For this review, use the dimensioned drawing (mm, ordinates from the lowest corner) and the shaded views. Round coordinates to 2 decimals unless told otherwise and drop trailing zeros. Loops run counter-clockwise (first coordinate to the right, second up) from the corner with the lowest first, then second, coordinate; pieces in that order, holes last. Notation, with made-up numbers: (33, 68) -> (82, 68) arc R16 cw to (82, 97) -> close; hole circle Ø1 at (86.25, 57.25). An arc over 180 degrees is marked (long way). Answer as CSV lines item,"result". Start each with the question number.
(1) Take a section at D-D, the plane y = 16.75. Write out the cut boundary in (x, z), and give its area (3 significant figures).
(2) For P1, Ø3, axis at y = 3, z = 1, coming from the +X side, flat-tipped, find the tip position at first contact; note if it passes through.
(3) Take a section at A-A, the plane y = 7.25. Write out the cut boundary in (x, z), and give its area (3 significant figures).
(4) Take a section at C-C, the plane z = 2.25. State how many separate pieces and enclosed holes the cut face has, and give its area (3 significant figures).
(5) Take a section at B-B, the plane x = 132. Write out the cut boundary in (y, z).
(6) To check wall thickness, follow line 1 (X direction, y = 9.25, z = 4.5); line 2 (X direction, y = 9, z = 0.75); line 3 (Y direction, x = 131.5, z = 3.5). State the ranges of each line that lie inside material, in increasing order. Write a range as from..to.
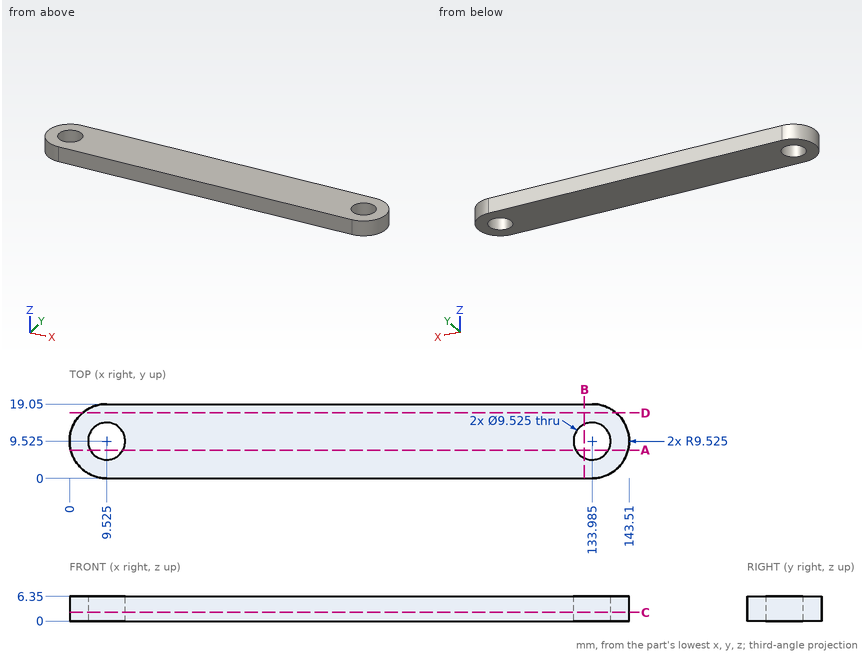
The answers:
1,outline,"(3.32, 0) -> (140.19, 0) -> (140.19, 6.35) -> (3.32, 6.35) -> close"
1,area,"869 mm²"
2,P1,"x = 142.08"
3,outline,"(0.28, 0) -> (5.34, 0) -> (5.34, 6.35) -> (0.28, 6.35) -> close; (13.71, 0) -> (129.8, 0) -> (129.8, 6.35) -> (13.71, 6.35) -> close; (138.17, 0) -> (143.23, 0) -> (143.23, 6.35) -> (138.17, 6.35) -> close"
3,area,"802 mm²"
4,separate pieces,"1"
4,enclosed holes,"2"
4,area,"2,510 mm²"
5,outline,"(0, 0) -> (5.2, 0) -> (5.2, 6.35) -> (0, 6.35) -> close; (13.85, 0) -> (19.05, 0) -> (19.05, 6.35) -> (13.85, 6.35) -> close"
6,line 1,"0..4.77, 14.28..129.23, 138.74..143.51"
6,line 2,"0.01..4.79, 14.26..129.25, 138.72..143.5"
6,line 3,"0..5.46, 13.59..19.05"
